The listing builds one solid part. Answer for the finished solid, in the listing's coordinates (mm). Face numbers are marked on the shaded views. A direction names the side the tool comes from. Give positions to 0.01 mm unless a question says otherwise; leave off trailing zeros. Order: outer loops, then holes, each group sorted by start corner. A loop starts at its lowest first (then second) coordinate and runs counter-clockwise, first axis right, second up. Notation, with made-up numbers: (52.5, 8.5) - (89.5, 8.5) arc R25 ccw to (89.5, 24.5) - close; hole circle Ø5 at (6, 83). An arc over 180 degrees is marked (long way). Write each question's results on one line, items separated by ' | '. Start each with the question number.
1. Section B-B (z = 8) is taken. Give the vertices of the cut face in (x, y).
2. Which of the six approach directions +Z, -Z, +X, -X, +Y, -Y give full straight-line access (tool end or side, diameter ignored) to the marked faces 4, 5, 6, 7 and 8?
3. Determine the mould class of the marked faces 1, 2 and 3 for opening direction X: released by +X, released by -X, zero draft, split by the parting line, or undercut.
4. Section A-A (y = -1.15) is taken. State how many separate pieces and enclosed holes the cut face has, and give its area (3 significant figures).
5. Find the intervals of material crossed by L1, parallel to Z at x = 22, y = -2.6; L2, parallel to X at y = -0.6, z = 50.5; L3, parallel to Z at x = 35, y = -2.35, in increasing order.
6. Flat-ended cylindrical pins translate along their axes: pin 1 (1.6 mm diameter, centred on x = 37.5, y = -1.5, fed in from +Z); pin 2 (0.9 mm diameter, centred on y = -3.5, z = 3.5, fed in from +X); pin 3 (1.5 mm diameter, centred on y = -2.5, z = 17, fed in from +X); pin 4 (8 mm diameter, centred on x = 10, z = 35, fed in from +Y). Find the tip coordinate at first contact, or state that the pin passes through.
7. Section C-C (x = 7) is taken. Give the vertices of the cut face in (y, z), and give its area (3 significant figures).
from build123d import *

# Parameters (mm, degrees)
F1_DEPTH = 5


with BuildPart() as f1:
    # F0 (on Front) → F1 (new body)
    with BuildSketch(Plane.XZ):
        Polygon((56.602631, 9.598027), (56.602631, 10.737107), (55.463549, 10.737107), (55.463549, 12.139052), (55.113062, 12.927647), (54.674953, 14.24197), (54.236848, 15.030565), (55.032882, 15.472803), (55.726416, 15.472803), (56.602631, 15.472803), (56.602631, 20.375481), (55.63879, 21.164075), (54.499712, 21.164075), (53.185388, 20.375481), (51.520579, 21.164075), (50.03101, 22.916507), (50.03101, 23.617478), (48.891932, 23.617478), (46.613768, 24.668938), (46.921512, 25.335718), (45.665746, 25.915302), (46.145314, 26.954366), (46.921512, 28.349044), (46.921512, 29.488124), (48.190959, 30.627204), (48.190959, 31.591043), (48.979554, 35.183527), (46.921512, 38.075037), (40.129773, 40.44082), (31.455237, 40.44082), (30.447589, 40.44082), (30.96698, 42.806929), (29.439941, 44.033308), (29.439941, 44.909522), (28.039239, 45.216994), (28.039239, 47.625791), (25.935078, 49.903952), (22.254972, 51.919248), (21.203512, 51.919248), (16.296705, 56.777831), (1.23168, 56.777831), (1.23168, 40.518545), (13.142328, 35.183527), (14.36903, 35.183527), (15.508111, 33.781581), (16.384326, 33.781581), (15.508111, 31.766284), (16.860185, 31.178426), (17.435785, 29.137637), (18.574866, 28.173801), (19.713946, 27.648071), (16.121462, 22.653641), (16.121462, 21.777425), (17.873893, 21.777425), (20.502539, 23.529857), (21.816865, 24.844181), (23.350241, 23.310802), (24.795998, 21.164075), (26.07753, 20.242271), (27.599888, 19.499265), (28.476104, 19.061157), (29.001834, 18.184941), (29.177075, 16.432509), (29.615184, 13.803862), (32.243829, 11.262836), (33.996262, 9.77327), (36.186803, 8.72181), (37.413504, 9.510404), (36.186803, 10.649486), (35.135344, 10.91235), (35.748694, 12.314295), (36.362045, 14.066727), (37.676368, 13.365754), (38.114477, 11.963809), (37.939236, 10.386621), (37.15064, 5.91792), (36.011558, 2.588299), (44.220895, 2.588299), (44.220895, 3.658485), (45.838311, 7.063572), (46.774711, 3.998994), (45.838311, 2.697169), (56.819715, 2.697169), align=None)
        Polygon((38.723323, 32.324277), (37.710983, 31.31194), (37.104577, 32.324277), align=None, mode=Mode.SUBTRACT)
        Polygon((35.48583, 34.657795), (38.723323, 34.652654), (38.723323, 33.336617), (35.48583, 33.336617), align=None, mode=Mode.SUBTRACT)
        Polygon((29.814744, 37.790902), (32.243829, 38.803242), (38.520854, 35.8845), align=None, mode=Mode.SUBTRACT)
        Polygon((41.557871, 37.588436), (40.849231, 36.474865), (39.53319, 36.272395), (34.1678, 38.803242), align=None, mode=Mode.SUBTRACT)
    extrude(amount=F1_DEPTH)


solid = f1.part
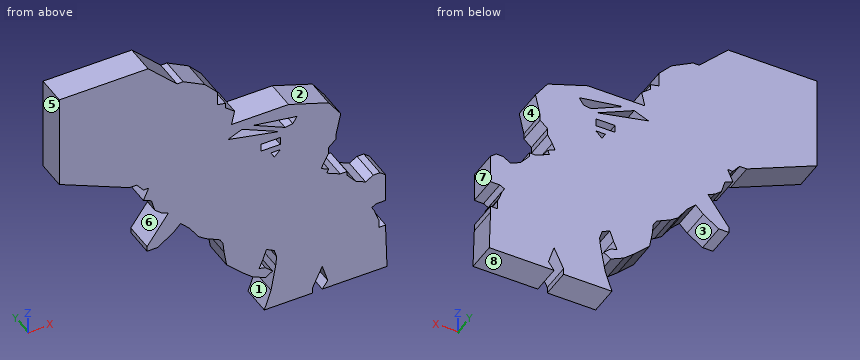
Reported:
1) outline: (37.52, -5) - (56.65, -5) - (56.65, 0) - (37.52, 0) - close
2) face 4: +X, +Y, -Y | face 5: +Z, -Z, -X, +Y, -Y | face 6: -X, +Y, -Y | face 7: +Z, +X, +Y, -Y | face 8: -Z, +X, +Y, -Y
3) face 1: released by -X | face 2: released by +X | face 3: undercut
4) separate pieces: 1 | enclosed holes: 4 | area: 1,420 mm²
5) L1: 24.66 to 51.92 | L2: 1.23 to 24.85 | L3: 9.29 to 36.66, 37.52 to 38.41, 38.67 to 40.44
6) pin 1: z = 40.44 | pin 2: x = 56.81 | pin 3: x = 56.6 | pin 4: y = 0
7) outline: (-5, 37.93) - (0, 37.93) - (0, 56.78) - (-5, 56.78) - close | area: 94.2 mm²
